CAD build for the part. Positions are in the model's coordinates, mm. A direction names the side the tool comes from. Give positions to 0.01 mm unless a question says otherwise; leave off trailing zeros. Order: outer loops, then holes, each group sorted by start corner. A loop starts at its lowest first (then second) coordinate and runs counter-clockwise, first axis right, second up. Notation, with made-up numbers: M 75.5,75 L 93.5,75 A34 cw 93.5,108 Z; hole C 12.25,57 d10. An arc over 180 degrees is marked long. Put each result on its own line as item: value. Start each with the question number.
1) Cut at D-D (x = 22). Write the cut outline in (y, z).
2) Tool access for faces 5 (the face through (-33, -15, 5)), 6 (the face through (34, -1, 4)), 7 (the face through (33, -15, 5)), 8 (the face through (33, 15, 5)), 9 (the face through (18, -19, 4)): list every direction of +Z, -Z, +X, -X, +Y, -Y with a clear straight run to the whole face (end or side of a thin tool).
3) Cut at C-C (y = 3.5). Write the cut outline in (x, z), and give its area (3 significant figures).
4) Pin check, flat tips, straight feed: pin 1 (3.5 mm diameter, centred on y = 18, z = 3.5, fed in from +X); pin 2 (0.8 mm diameter, centred on x = -32.5, z = 7, fed in from +Y); pin 3 (3.5 mm diameter, centred on x = -33, y = 13, fed in from -Z); pin 4 (20 mm diameter, centred on x = 0.5, y = -5, fed in from -Z). Stop position of each tip, or through.
5) Two-plate mould, pull along X, no slides. Class faces 1 (the face through (-30, 19, 5)), 2 (the face through (28, -17, 4)), 3 (the face through (33.508, 12.024, 4.93)), 4 (the face through (32, -10, 0)): released by +X, released by -X, zero draft, split by the parting line, or undercut.
6) Drill centre lines: line 1 (Y direction, x = -3.5, z = 5); line 2 (X direction, y = 13, z = 4); line 3 (Z direction, x = -10, y = 4). Where is each one in solid material? Low to high. Write a range as [from, to].
7) Cut at B-B (x = -9). Write the cut outline in (y, z).
8) Cut at A-A (z = 8.75). Write the cut outline in (x, y), and give its area (3 significant figures).
```python
from build123d import *

# Parameters (mm, degrees)
PAD_DEPTH       = 10
SKETCH002_R     = 1.1
HOLE_DEPTH      = 25
POCKET001_DEPTH = 8
SKETCH004_W     = 8
SKETCH004_H     = 4
SKETCH004_W_2   = 10
SKETCH004_W_3   = 4
SKETCH004_H_2   = 10
POCKET002_DEPTH = 8
FILLET_R        = 1.5


with BuildPart() as part:
    # Sketch → Pad (new body)
    with BuildSketch(Plane.XY):
        with BuildLine():
            ThreePointArc((-30, -17), (-30.585786, -15.585786), (-32, -15))
            Line((-32, -15), (-35, -15))
            Line((-35, 15), (-35, -15))
            Line((-32, 15), (-35, 15))
            ThreePointArc((-32, 15), (-30.585786, 15.585786), (-30, 17))
            Line((-30, 20), (-30, 17))
            Line((30, 20), (-30, 20))
            Line((30, 20), (30, 17))
            ThreePointArc((30, 17), (30.585786, 15.585786), (32, 15))
            Line((32, 15), (35, 15))
            Line((35, 15), (35, -15))
            Line((32, -15), (35, -15))
            ThreePointArc((32, -15), (30.585786, -15.585786), (30, -17))
            Line((30, -17), (30, -20))
            Line((-30, -20), (30, -20))
            Line((-30, -17), (-30, -20))
        make_face()
    extrude(amount=PAD_DEPTH)

    # Sketch002 → Hole (cut)
    with BuildSketch(Plane.XY):
        with Locations((33, 13)):
            Circle(SKETCH002_R)
        with Locations((33, -13)):
            Circle(SKETCH002_R)
        with Locations((-33, -13)):
            Circle(SKETCH002_R)
        with Locations((-33, 13)):
            Circle(SKETCH002_R)
    extrude(amount=HOLE_DEPTH, mode=Mode.SUBTRACT)

    # Sketch003 → Pocket001 (cut)
    with BuildSketch(Plane.XY):
        with BuildLine():
            Line((28, -18), (-28, -18))
            Line((-28, -18), (-28, -14))
            ThreePointArc((-28, -14), (-29.464466, -10.464466), (-33, -9))
            Line((-33, -9), (-33, 9))
            ThreePointArc((-33, 9), (-29.464466, 10.464466), (-28, 14))
            Line((-28, 14), (-28, 18))
            Line((-28, 18), (28, 18))
            Line((28, 18), (28, 14))
            ThreePointArc((28, 14), (29.464466, 10.464466), (33, 9))
            Line((33, 9), (33, -9))
            ThreePointArc((33, -9), (29.464466, -10.464466), (28, -14))
            Line((28, -14), (28, -18))
        make_face()
    extrude(amount=POCKET001_DEPTH, mode=Mode.SUBTRACT)

    # Sketch004 → Pocket002 (cut)
    with BuildSketch(Plane.XY):
        with Locations((-24, 19)):
            Rectangle(SKETCH004_W, SKETCH004_H)
        with Locations((23, -19)):
            Rectangle(SKETCH004_W_2, SKETCH004_H)
        with Locations((34, 4)):
            Rectangle(SKETCH004_W_3, SKETCH004_H_2)
    extrude(amount=POCKET002_DEPTH, mode=Mode.SUBTRACT)

    # Fillet
    fillet_edges = [part.edges().sort_by_distance(p)[0] for p in [
        (35, -15, 5),
        (35, 15, 5),
        (-35, -15, 5),
        (-35, 15, 5),
    ]]
    fillet(fillet_edges, radius=FILLET_R)


solid = part.part
```
Solution:
1. outline: M -20,8 L 18,8 L 18,0 L 20,0 L 20,10 L -20,10 Z
2. face 5: +Z, -Z, -X, -Y
2. face 6: -Z, +X
2. face 7: +Z, -Z, +X, -Y
2. face 8: +Z, -Z, +X, +Y
2. face 9: -Z, -Y
3. outline: M -35,0 L -33,0 L -33,8 L 35,8 L 35,10 L -35,10 Z
3. area: 156 mm²
4. pin 1: x = 30.15
4. pin 2: y = 15
4. pin 3: z = 0
4. pin 4: z = 8
5. face 1: released by -X
5. face 2: undercut
5. face 3: undercut
5. face 4: zero draft
6. line 1: [-20, -18], [18, 20]
6. line 2: [-35, -34.1], [-31.9, -28.1], [28.1, 31.9], [34.1, 35]
6. line 3: [8, 10]
7. outline: M -20,0 L -18,0 L -18,8 L 18,8 L 18,0 L 20,0 L 20,10 L -20,10 Z
8. outline: M -35,-13.5 A1.5 ccw -33.5,-15 L -32,-15 A2 cw -30,-17 L -30,-20 L 30,-20 L 30,-17 A2 cw 32,-15 L 33.5,-15 A1.5 ccw 35,-13.5 L 35,13.5 A1.5 ccw 33.5,15 L 32,15 A2 cw 30,17 L 30,20 L -30,20 L -30,17 A2 cw -32,15 L -33.5,15 A1.5 ccw -35,13.5 Z; hole C -33,-13 d2.2; hole C -33,13 d2.2; hole C 33,-13 d2.2; hole C 33,13 d2.2
8. area: 2,690 mm²
